Source: three-view drawing plus pictorial views. Frame: mm from the lowest corner of the part. A direction names the side the tool comes from. Give positions to 0.01 mm unless a question says otherwise; leave off trailing zeros. Order: outer loops, then holes, each group sorted by start corner. A loop starts at its lowest first (then second) coordinate and runs counter-clockwise, first axis right, second up.
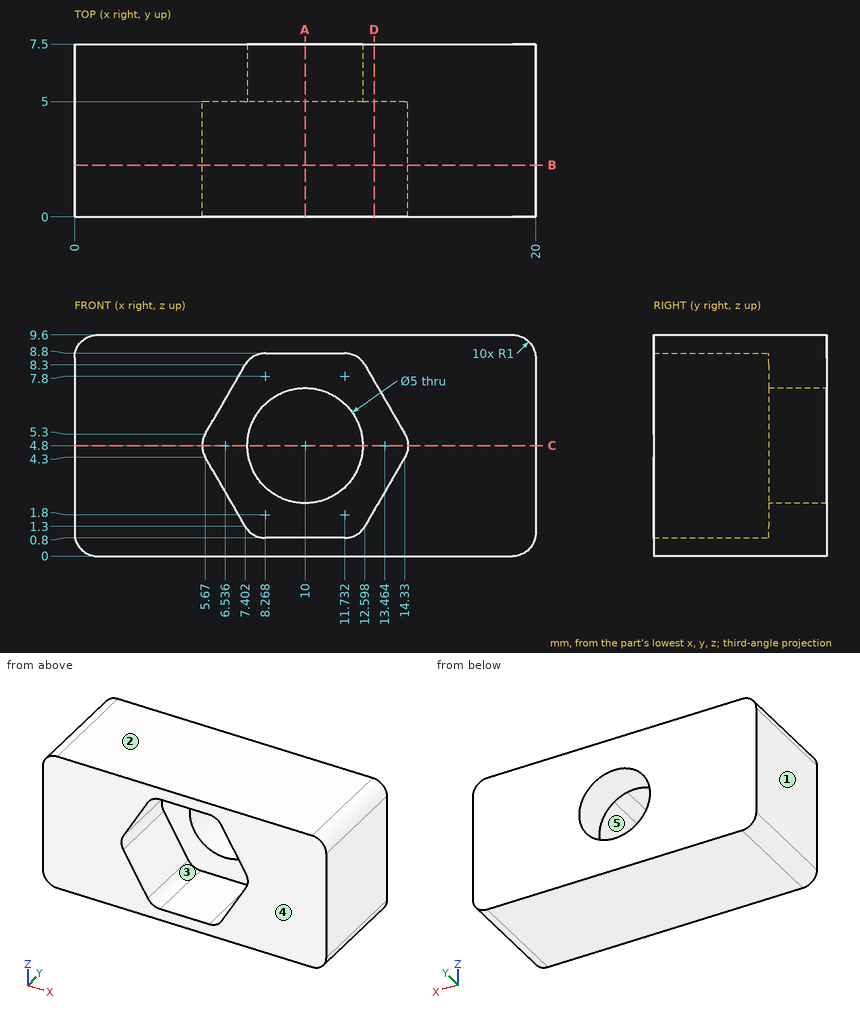
1) Section query C-C on z = 4.8. Output: boundary loops of the cut face in (x, y).
Checks:
outline: (0, 0) - (5.54, 0) - (5.54, 5) - (7.5, 5) - (7.5, 7.5) - (0, 7.5) - close; (12.5, 5) - (14.46, 5) - (14.46, 0) - (20, 0) - (20, 7.5) - (12.5, 7.5) - close
2) First-contact query: pin 1 Ø1.7 at (x, y) = (10.5, 2.5) entering from -Z; pin 2 Ø2.5 at (x, z) = (10.5, 3) entering from -Y. Flat tips, straight axial feed; report the tip coordinate or a pass-through.
Checks:
pin 1: stops at z = 0
pin 2: stops at y = 5
3) Reachability of the marked faces 4 and 5 from +Z, -Z, +X, -X, +Y, -Y: full face, straight path, thin tool, end or side. Return the list, or none.
Checks:
face 4: +Z, -Z, +X, -X, -Y
face 5: -Y
4) Section query D-D on x = 13. Output: boundary loops of the cut face in (y, z), and give its area (3 significant figures).
Checks:
outline: (0, 0) - (7.5, 0) - (7.5, 9.6) - (0, 9.6) - (0, 7.6) - (5, 7.6) - (5, 2) - (0, 2) - close
area: 44.0 mm2
5) Pull-direction query (Z, two-part tool) for the marked faces 1, 2 and 3; classes: +Z half, -Z half, draft (parallel to the pull), parting line (faces both ways), or undercut.
Checks:
face 1: draft
face 2: +Z half
face 3: undercut
6) Section query A-A on x = 10. Output: boundary loops of the cut face in (y, z).
Checks:
outline: (0, 0) - (7.5, 0) - (7.5, 2.3) - (5, 2.3) - (5, 0.8) - (0, 0.8) - close; (0, 8.8) - (5, 8.8) - (5, 7.3) - (7.5, 7.3) - (7.5, 9.6) - (0, 9.6) - close
7) Section query B-B on y = 2.25. Output: boundary loops of the cut face in (x, z).
Checks:
outline: (0, 1) arc R1 ccw to (1, 0) - (19, 0) arc R1 ccw to (20, 1) - (20, 8.6) arc R1 ccw to (19, 9.6) - (1, 9.6) arc R1 ccw to (0, 8.6) - close; hole (5.67, 4.3) - (7.4, 1.3) arc R1 ccw to (8.27, 0.8) - (11.73, 0.8) arc R1 ccw to (12.6, 1.3) - (14.33, 4.3) arc R1 ccw to (14.33, 5.3) - (12.6, 8.3) arc R1 ccw to (11.73, 8.8) - (8.27, 8.8) arc R1 ccw to (7.4, 8.3) - (5.67, 5.3) arc R1 ccw to start
8) Ray query, L1, parallel to X at y = 5.9, z = 4.8; L2, parallel to X at y = 2.75, z = 4.75; L3, parallel to Z at x = 14, y = 2. Return the intervals inside material, ascending.
Checks:
L1: x = 0 to 7.5, 12.5 to 20
L2: x = 0 to 5.54, 14.46 to 20
L3: z = 0 to 3.73, 5.87 to 9.6
